from build123d import *

# Parameters (mm, degrees)
EXTRUDE_1_DEPTH     = 360
SKETCH_2_R          = 1.5
CUT_EXTRUDE_1_DEPTH = 380


with BuildPart() as part:
    # 草图1 → 凸台-拉伸1 (new body)
    with BuildSketch(Plane.XY):
        Polygon((0, 0), (0, 180), (-1, 180), (-1, 0.363970234), (-13.621796637, -14.678101253), (-12.855752194, -15.320888862), align=None)
    extrude(amount=EXTRUDE_1_DEPTH)

    # 草图2 → 切除-拉伸1 (cut)
    with BuildSketch(Plane.ZY.offset(1)):
        with Locations((305.5, 31.363970234)):
            Circle(SKETCH_2_R)
        with Locations((305.5, 43.363970234)):
            Circle(SKETCH_2_R)
        with Locations((305.5, 121.363970234)):
            Circle(SKETCH_2_R)
        with Locations((305.5, 133.363970234)):
            Circle(SKETCH_2_R)
        with Locations((54.5, 121.363970234)):
            Circle(SKETCH_2_R)
        with Locations((54.5, 31.363970234)):
            Circle(SKETCH_2_R)
        with Locations((54.5, 43.363970234)):
            Circle(SKETCH_2_R)
        with Locations((54.5, 133.363970234)):
            Circle(SKETCH_2_R)
    extrude(amount=-CUT_EXTRUDE_1_DEPTH, mode=Mode.SUBTRACT)


solid = part.part
Read the model definition and answer for the solid it produces. Units are mm, in the model's axes. A direction names the side the tool comes from. Give positions to 0.01 mm unless a question says otherwise; leave off trailing zeros. Write each loop counter-clockwise with the first axis right and the second up, starting at its lowest first coordinate (ties: lowest second). Pieces come first, ordered by that corner, then holes. Notation, with made-up numbers: (39, 34.25) - (79, 34.25) arc R17 ccw to (79, 50.25) - close; hole circle Ø8 at (80, -7). An arc over 180 degrees is marked (long way). Answer in a Markdown table with one row per item. Add a question column.
Item 1: Flat-ended cylindrical pins translate along their axes: P1, Ø5, axis at x = -2.5, z = 310, coming from the -Y side; P2, Ø4, axis at y = 98, z = 285, coming from the -X side; P3, Ø5, axis at x = -5, z = 132.5, coming from the +Y side. Find the tip coordinate at first contact, or state that the pin passes through.
Item 2: Section C-C, the plane x = -9.5 is taken. Write down the section's boundary in (y, z), and give its area (3 significant figures).
Item 3: A tool of negligible diameter and unlimited length cuts with its end or side. For faces 1 (the face through (-1, 91, 177)), 2 (the face through (-0.8, 82.8, 0)), from which of +Z, -Z, +X, -X, +Y, -Y can it reach the whole face along a straight path? Write none if from no direction.
Item 4: Section B-B, the plane y = 83 is taken. Write down the section's boundary in (x, z), and give its area (3 significant figures).
Item 5: Section A-A, the plane z = 141 is taken. Write down the section's boundary in (x, y).
Item 6: Find the intervals of material crossed by L1, parallel to Y at x = -0.65, z = 54.5; L2, parallel to Y at x = -0.4, z = 305.5; L3, parallel to X at y = 49.5, z = 344, in increasing order.
Recorded:
| question | item | result |
|---|---|---|
| 1 | P1 | stops at y = -5.96 |
| 1 | P2 | stops at x = -1 |
| 1 | P3 | stops at y = -1.42 |
| 2 | outline | (-11.32, 0) - (-9.77, 0) - (-9.77, 360) - (-11.32, 360) - close |
| 2 | area | 560 mm2 |
| 3 | face 1 | +Z, -Z, -X, +Y |
| 3 | face 2 | -Z, +X, -X, +Y, -Y |
| 4 | outline | (-1, 0) - (0, 0) - (0, 360) - (-1, 360) - close |
| 4 | area | 360 mm2 |
| 5 | outline | (-13.62, -14.68) - (-12.86, -15.32) - (0, 0) - (0, 180) - (-1, 180) - (-1, 0.36) - close |
| 6 | L1 | y = -0.77 to 29.86, 32.86 to 41.86, 44.86 to 119.86, 122.86 to 131.86, 134.86 to 180 |
| 6 | L2 | y = -0.48 to 29.86, 32.86 to 41.86, 44.86 to 119.86, 122.86 to 131.86, 134.86 to 180 |
| 6 | L3 | x = -1 to 0 |
